```python
from build123d import *

# Parameters (mm, degrees)
SKETCH2_W           = 34.99
SKETCH2_H           = 7.1
SKETCH2_R           = 1.525
BOSS_EXTRUDE1_DEPTH = 3
SKETCH3_W           = 34.99
SKETCH3_H           = 2
BOSS_EXTRUDE2_DEPTH = 6
SKETCH4_W           = 7
SKETCH4_H           = 7
BOSS_EXTRUDE3_DEPTH = 60
SKETCH5_W           = 34.99
SKETCH5_H           = 11.1
SKETCH5_R           = 1.525
BOSS_EXTRUDE4_DEPTH = 2.5


with BuildPart() as part:
    # Sketch2 → Boss-Extrude1 (new body)
    with BuildSketch(Plane.XY):
        with Locations((13.97, 0)):
            Rectangle(SKETCH2_W, SKETCH2_H)
        Circle(SKETCH2_R, mode=Mode.SUBTRACT)
        with Locations((27.94, 0)):
            Circle(SKETCH2_R, mode=Mode.SUBTRACT)
    extrude(amount=BOSS_EXTRUDE1_DEPTH)

    # Sketch3 → Boss-Extrude2 (add)
    with BuildSketch(Plane.XY.offset(3)):
        with Locations((13.97, -4.55)):
            Rectangle(SKETCH3_W, SKETCH3_H)
        with Locations((13.97, 4.55)):
            Rectangle(SKETCH3_W, SKETCH3_H)
    extrude(amount=-BOSS_EXTRUDE2_DEPTH)

    # Sketch4 → Boss-Extrude3 (add)
    with BuildSketch(Plane.XY.offset(3)):
        with Locations((13.97, 0)):
            Rectangle(SKETCH4_W, SKETCH4_H)
    extrude(amount=BOSS_EXTRUDE3_DEPTH)

    # Sketch5 → Boss-Extrude4 (add)
    with BuildSketch(Plane.XY.offset(63)):
        with Locations((13.97, 0)):
            Rectangle(SKETCH5_W, SKETCH5_H)
        Circle(SKETCH5_R, mode=Mode.SUBTRACT)
        with Locations((27.94, 0)):
            Circle(SKETCH5_R, mode=Mode.SUBTRACT)
    extrude(amount=BOSS_EXTRUDE4_DEPTH)


solid = part.part
```
Model file for the job. Use its own axes, mm. A direction names the side the tool comes from. Coordinates: 2 decimals unless noted, no trailing zeros. Write each loop counter-clockwise with the first axis right and the second up, starting at its lowest first coordinate (ties: lowest second). Pieces come first, ordered by that corner, then holes. Notation, with made-up numbers: (69.5, -29) - (125.5, -29) arc R30 ccw to (125.5, 3) - close; hole circle Ø9 at (6, 22.5). An arc over 180 degrees is marked (long way). Use a Markdown table: item, result. Add a question column.
Item 1: 3-axis set-ups, long thin cutter, end or side, ignore diameter. For faces 1 (the face through (14, -3.5, 33)), 2 (the face through (10.47, 0, 33)), 3 (the face through (14, 0, 0)): which of +Z, -Z, +X, -X, +Y, -Y reach the whole face in a straight line?
Item 2: Band-saw the part on A-A, the plane x = 25. Write the cut outline in (y, z), and give its area (4 significant figures).
Item 3: Two-plate mould, pull along Y, no slides. Class faces 4 (the face through (14, 5.55, 0)), 5 (the face through (-1.524, 0.067, 64.232)), 6 (the face through (14, -5, -3)): pulls with the +Y half, pulls with the -Y half, needs draft (parallel to the pull), parting line crosses it, or undercut.
Item 4: Drop flat-ended pins along their axis: pin 1 (3 mm diameter, centred on y = -2, z = 43, fed in from +X); pin 2 (3.5 mm diameter, centred on x = 18, y = -1.5, fed in from -Z); pin 3 (4 mm diameter, centred on x = 15.5, z = 39.5, fed in from -Y). Give the stop position or say it passes through.
Item 5: Band-saw the part on D-D, the plane z = 51. Write the cut outline in (x, y).
Item 6: Band-saw the part on C-C, the plane x = 12. Write the cut outline in (y, z).
Item 7: Drill centre lines: line 1 along Z through (x, y) = (2, -0.5); line 2 along Z through (x, y) = (16, 4.5); line 3 along Y through (x, z) = (0, 64.2) (3 decimals). Where is each one in solid material? Low to high.
Item 8: Band-saw the part on B-B, the plane y = 0. Write the cut outline in (x, z) (3 decimals), and give its area (3 significant figures).
A:
| question | item | result |
|---|---|---|
| 1 | face 1 | +X, -X, -Y |
| 1 | face 2 | -X, +Y, -Y |
| 1 | face 3 | -Z, +X, -X |
| 2 | outline | (-5.55, -3) - (-3.55, -3) - (-3.55, 0) - (3.55, 0) - (3.55, -3) - (5.55, -3) - (5.55, 3) - (-5.55, 3) - close; (-5.55, 63) - (5.55, 63) - (5.55, 65.5) - (-5.55, 65.5) - close |
| 2 | area | 73.05 mm² |
| 3 | face 4 | pulls with the +Y half |
| 3 | face 5 | undercut |
| 3 | face 6 | needs draft |
| 4 | pin 1 | stops at x = 17.47 |
| 4 | pin 2 | stops at z = 0 |
| 4 | pin 3 | stops at y = -3.5 |
| 5 | outline | (10.47, -3.5) - (17.47, -3.5) - (17.47, 3.5) - (10.47, 3.5) - close |
| 6 | outline | (-5.55, -3) - (-3.55, -3) - (-3.55, 0) - (3.55, 0) - (3.55, -3) - (5.55, -3) - (5.55, 3) - (3.5, 3) - (3.5, 63) - (5.55, 63) - (5.55, 65.5) - (-5.55, 65.5) - (-5.55, 63) - (-3.5, 63) - (-3.5, 3) - (-5.55, 3) - close |
| 7 | line 1 | z = 0 to 3, 63 to 65.5 |
| 7 | line 2 | z = -3 to 3, 63 to 65.5 |
| 7 | line 3 | y = -5.55 to -1.525, 1.525 to 5.55 |
| 8 | outline | (-3.525, 0) - (-1.525, 0) - (-1.525, 3) - (-3.525, 3) - close; (-3.525, 63) - (-1.525, 63) - (-1.525, 65.5) - (-3.525, 65.5) - close; (1.525, 0) - (26.415, 0) - (26.415, 3) - (17.47, 3) - (17.47, 63) - (26.415, 63) - (26.415, 65.5) - (1.525, 65.5) - (1.525, 63) - (10.47, 63) - (10.47, 3) - (1.525, 3) - close; (29.465, 0) - (31.465, 0) - (31.465, 3) - (29.465, 3) - close; (29.465, 63) - (31.465, 63) - (31.465, 65.5) - (29.465, 65.5) - close |
| 8 | area | 579 mm² |
